Geometry: final body of the model. Coordinates: model frame, mm. Give positions to 0.01 mm unless a question says otherwise; leave off trailing zeros. Loops run counter-clockwise (first coordinate to the right, second up) from the corner with the lowest first, then second, coordinate; pieces in that order, holes last. Notation, with made-up numbers: (34.25, 5) -> (73.25, 5) arc R31 cw to (73.25, 38) -> close; hole circle Ø11 at (40, 79). An arc over 180 degrees is marked (long way). Answer in a Markdown table with one row per item. Add a question column.
from build123d import *

# Parameters (mm, degrees)
CROQUIS1_R              = 11
SALIENTE_EXTRUIR1_DEPTH = 5


with BuildPart() as part:
    # Croquis1 → Saliente-Extruir1 (new body)
    with BuildSketch(Plane.XY):
        with BuildLine():
            Line((-13.747727085, 81), (-41.243181255, 18))
            ThreePointArc((-41.243181255, 18), (0, -45), (41.243181255, 18))
            Line((41.243181255, 18), (13.747727085, 81))
            ThreePointArc((13.747727085, 81), (0, 90), (-13.747727085, 81))
        make_face()
        with Locations((0, 75)):
            Circle(CROQUIS1_R, mode=Mode.SUBTRACT)
        with BuildLine():
            ThreePointArc((24.748737342, -24.748737342), (0, 35), (-24.748737342, -24.748737342))
            ThreePointArc((-24.748737342, -24.748737342), (-10.606601718, -24.748737342), (-10.606601718, -10.606601718))
            ThreePointArc((-10.606601718, -10.606601718), (0, 15), (10.606601718, -10.606601718))
            ThreePointArc((10.606601718, -10.606601718), (10.606601718, -24.748737342), (24.748737342, -24.748737342))
        make_face(mode=Mode.SUBTRACT)
    extrude(amount=SALIENTE_EXTRUIR1_DEPTH)


solid = part.part
(1) Cut plane C-C on y = 23. Return the cut outline in (x, z).
(2) Cut plane B-B on y = 0. Return the cut outline in (x, z), then the cut area to 3 significant figures.
(3) Cut plane A-A on x = 0. Return the cut outline in (y, z).
(4) Draft query along X for faces 1 (the cylindrical face through (0, 90, 2)), 2 (the cylindrical face through (-10.76, -24.9, 2.46)), 3 (the flat face through (-27.303, 49.941, 2.465)). Return one class per face: +X half, -X half, draft (parallel to the pull), parting line (faces both ways), or undercut.
(5) Pin query (flat end, axial travel): pin 1 Ø10 at (x, y) = (-26.5, 0.5) entering from +Z. Return the tip coordinate at first contact, or that it passes through.
(6) Material intervals for line 1 along Y through (x, z) = (-0.5, 1.15); line 2 along Y through (x, z) = (10, 1.35); line 3 along Y through (x, z) = (-7, 1.85), sorted ascending. Write a range as from..to.
(7) Cut plane D-D on z = 3.05. Return the cut outline in (x, y), then the cut area to 3 significant figures.
Answer list:
| question | item | result |
|---|---|---|
| 1 | outline | (-39.06, 0) -> (-26.38, 0) -> (-26.38, 5) -> (-39.06, 5) -> close; (26.38, 0) -> (39.06, 0) -> (39.06, 5) -> (26.38, 5) -> close |
| 2 | outline | (-45, 0) -> (-35, 0) -> (-35, 5) -> (-45, 5) -> close; (-15, 0) -> (15, 0) -> (15, 5) -> (-15, 5) -> close; (35, 0) -> (45, 0) -> (45, 5) -> (35, 5) -> close |
| 2 | area | 250 mm² |
| 3 | outline | (-45, 0) -> (15, 0) -> (15, 5) -> (-45, 5) -> close; (35, 0) -> (64, 0) -> (64, 5) -> (35, 5) -> close; (86, 0) -> (90, 0) -> (90, 5) -> (86, 5) -> close |
| 4 | face 1 | parting line |
| 4 | face 2 | undercut |
| 4 | face 3 | -X half |
| 5 | pin 1 | passes through |
| 6 | line 1 | y = -45..14.99, 35..64.01, 85.99..89.99 |
| 6 | line 2 | y = -43.87..-24.08, -11.27..11.18, 33.54..70.42, 79.58..86.18 |
| 6 | line 3 | y = -44.45..13.27, 34.29..66.51, 83.49..88.27 |
| 7 | outline | (-41.24, 18) arc R45 ccw (long way) to (41.24, 18) -> (13.75, 81) arc R15 ccw to (-13.75, 81) -> close; hole (-24.75, -24.75) arc R10 ccw to (-10.61, -10.61) arc R15 cw (long way) to (10.61, -10.61) arc R10 ccw to (24.75, -24.75) arc R35 ccw (long way) to start; hole circle Ø22 at (0, 75) |
| 7 | area | 5,350 mm² |
